```python
from build123d import *

# Parameters (mm, degrees)
F0_W      = 12
F0_H      = 64
F1_DEPTH  = 24
F2_DEPTH  = 65
F3_W      = 24
F3_H      = 24
F4_DEPTH  = 20
F6_DEPTH  = 37.6
F8_DEPTH  = 41
F9_W      = 44
F9_H      = 44
F10_DEPTH = 12
F11_W     = 44
F11_H     = 44
F12_DEPTH = 53
F14_DEPTH = 44


with BuildPart() as f1:
    # F0 (on Top) → F1 (new body)
    with BuildSketch(Plane.XY):
        with Locations((38, 0)):
            Rectangle(F0_W, F0_H)
    extrude(amount=F1_DEPTH)

    # F0 (on Top) → F2 (join)
    with BuildSketch(Plane.XY):
        Polygon((32, -32), (32, 32), (-44, 32), (-44, 12), (0, 12), (0, -32), align=None)
    extrude(amount=F2_DEPTH)

    # F3 (on face) → F4 (join)
    with BuildSketch(Plane.YZ.offset(44)):
        with Locations((0, 12)):
            Rectangle(F3_W, F3_H)
    extrude(amount=F4_DEPTH)

    # F5 (on face) → F6 (cut)
    with BuildSketch(Plane.XZ.offset(12)):
        Polygon((64, 24), (49.7921183705, 24), (64, 0), align=None)
    extrude(amount=-F6_DEPTH, mode=Mode.SUBTRACT)

    # F7 (on face) → F8 (cut)
    with BuildSketch(Plane.XY.offset(65)):
        with BuildLine():
            ThreePointArc((32, 20), (12, 0), (32, -20))
            Line((32, -20), (32, 20))
        make_face()
    extrude(amount=-F8_DEPTH, mode=Mode.SUBTRACT)

    # F9 (on face) → F10 (join)
    with BuildSketch(Plane.XY):
        with Locations((-22, -10)):
            Rectangle(F9_W, F9_H)
    extrude(amount=F10_DEPTH)

    # F11 (on face) → F12 (join)
    with BuildSketch(Plane.XY.offset(12)):
        with Locations((-22, -10)):
            Rectangle(F11_W, F11_H)
    extrude(amount=F12_DEPTH)

    # F13 (on face) → F14 (cut)
    with BuildSketch(Plane(origin=(-44, 0, 0), x_dir=(0, -1, 0), z_dir=(-1, 0, 0))):
        with BuildLine():
            Line((32, 65), (-12, 65))
            ThreePointArc((-12, 65), (0.8873016278, 33.8873016278), (32, 21))
            Line((32, 21), (32, 65))
        make_face()
    extrude(amount=-F14_DEPTH, mode=Mode.SUBTRACT)


solid = f1.part
```
The model under review builds one solid part; all positions refer to its coordinate system, in mm. A direction names the side the tool comes from. Round coordinates to 2 decimals unless told otherwise and drop trailing zeros. Write each loop counter-clockwise with the first axis right and the second up, starting at its lowest first coordinate (ties: lowest second). Pieces come first, ordered by that corner, then holes. Notation, with made-up numbers: (51, -35) - (62, -35) arc R19 cw to (62, -22) - close; hole circle Ø3 at (56, 30.25). An arc over 180 degrees is marked (long way). Answer as CSV lines item,"result". Start each with the question number.
(1) We need section B-B on y = -22.5. State the section outline as (x, z) points.
(2) Draft analysis for pull direction Y (two halves, no side actions). For faces 5 (the flat face through (52, 12, 9)), 6 (the flat face through (52, -12, 9)), 7 (the cylindrical face through (12, 0, 45)), 8 (the flat face through (32, 26, 44)), state which applies: pulls with the +Y half, pulls with the -Y half, needs draft (parallel to the pull), parting line crosses it, or undercut.
(3) For pin 1 Ø10 at (y, z) = (26.5, 16) entering from +X; pin 2 Ø13 at (y, z) = (-2, 37) entering from -X; pin 3 Ø1.5 at (x, y) = (-22.5, -10.5) entering from +Z; pin 4 Ø3 at (x, y) = (-28, -6) entering from +Z, all flat-tipped, find the tip position at first contact; note any pin that passes through.
(4) We need section A-A on z = 36. State the section outline as (x, y) points, plus the area to 3 significant figures.
(5) To check wall thickness, follow line 1 (Z direction, x = 16, y = -11.5); line 2 (X direction, y = 22, z = 13); line 3 (X direction, y = -28.5, z = 32). State the ranges of each line that lie inside material, in increasing order.
(6) For faces 1 (the flat face through (32, -26, 44)), 2 (the flat face through (44, -22, 12)), 3 (the flat face through (44, 22, 12)), 4 (the flat face through (0, -15, 48)), list the 3-axis set-ups (+Z, -Z, +X, -X, +Y, -Y) from which the entire face can be reached by the end or side of a thin tool; tool diameter is ignored.
(7) We need section C-C on x = 48. State the section outline as (y, z) points.
Worked answers:
1,outline,"(-44, 0) - (44, 0) - (44, 24) - (32, 24) - (32, 65) - (0, 65) - (0, 22.04) - (-44, 22.04) - close"
2,face 5,"pulls with the +Y half"
2,face 6,"pulls with the -Y half"
2,face 7,"undercut"
2,face 8,"needs draft"
3,pin 1,"x = 44"
3,pin 2,"x = -44"
3,pin 3,"z = 27.04"
3,pin 4,"z = 30.65"
4,outline,"(-44, 1.09) - (0, 1.09) - (0, -32) - (32, -32) - (32, -20) arc R20 cw to (32, 20) - (32, 32) - (-44, 32) - close"
4,area,"2,780 mm²"
5,line 1,"0 to 24"
5,line 2,"-44 to 44"
5,line 3,"0 to 32"
6,face 1,"+Z, +X, +Y, -Y"
6,face 2,"+Z, -Z, +X, -Y"
6,face 3,"+Z, -Z, +X, +Y"
6,face 4,"+Z, -X, -Y"
7,outline,"(-12, 0) - (12, 0) - (12, 24) - (-12, 24) - close"
